Can you work these out from the model? Positions are in its coordinate system, mm. A direction names the side the tool comes from. Round coordinates to 2 decimals unless told otherwise and drop trailing zeros. Loops run counter-clockwise (first coordinate to the right, second up) from the corner with the lowest first, then second, coordinate; pieces in that order, holes last. Notation, with made-up numbers: (-38.75, 70) -> (-15.75, 70) arc R21 ccw to (-15.75, 83) -> close; hole circle Ø7 at (27.5, 49.25). An arc over 180 degrees is marked (long way). Write item = value, one per line.
Autodesk Inventor part; units mm, degrees
ref_plane "YZ Plane" through (0, 0, 0) normal (1, 0, 0) x (0, 1, 0)
ref_plane "XZ Plane" through (0, 0, 0) normal (0, 1, 0) x (-1, 0, 0)
ref_plane "XY Plane" through (0, 0, 0) normal (0, 0, 1) x (1, 0, 0)
sketch "Sketch1" plane through (0, 0, 0) normal (0, 0, 1) x (1, 0, 0)
  line L0 (0, 0) -> (-50, 0) construction
  line L1 (-50, 0) -> (-50, 10)
  line L2 (-50, 0) -> (-50, -10)
  line L3 (-50, -10) -> (-30, -10)
  line L4 (-30, -10) -> (15, -37.5)
  line L5 (-50, 10) -> (-30, 10)
  line L6 (-30, 10) -> (15, 37.5)
  line L7 (15, 37.5) -> (15, -37.5)
  line L8 (0, 0) -> (15, 0) construction
  line L9 (0, 17.5) -> (0, -17.5) construction
  line L10 (-30, 10) -> (40, 10)
  line L11 (-30, -10) -> (40, -10)
  line L12 (40, 10) -> (40, -10)
  circle A0 centre (35, 0) radius 2.25
  circle A1 centre (15, 0) radius 2.25
  line L13 (35, 2.25) -> (15, 2.25)
  line L14 (15, -2.25) -> (35, -2.25)
  point P0 (-40, 0)
  point P1 (40, 0)
  point P2 (15, -10)
  point P3 (15, 10)
  point P4 (-20, 0)
  dimension "d0" = 20
  dimension "d1" = 65
  dimension "d2" = 50
  dimension "d4" = 20
  dimension "d5" = 75
  dimension "d6" = 35
  dimension "d9" = 40
  dimension "d21" = 25
  dimension "d22" = 5
  dimension "d23" = 4.5
  dimension "d30" = 20
extrude "Extrusion1" add sketch "Sketch1" along normal blind 5 contours L1 L5 L10 L7 A1 L11 L3 L2 | L6 L7 L10 | L11 L7 L4 | L7 A1 picked at (13.9746, 0.6255)
hole "Hole1" at (0, 17.5, 0) at (0, -17.5, 0) at (-40, 0, 0) at (0, 0, 0) at (-20, 0, 0) direction (0, 0, 1) diameter 4.5 end through all counterbore diameter 8 counterbore depth 2
fillet "Fillet1" radius 20 2 edges at (-30, 10, 2.5) (-30, -10, 2.5)
chamfer "Chamfer1" distance 2 angle 45 2 edges at (-50, 10, 2.5) (-50, -10, 2.5)
chamfer "Chamfer3" distance 4 angle 45 4 edges at (-5.0992, 25.2172, 0) (-41.8137, 10, 0) (-41.8137, -10, 0) (-5.0992, -25.2172, 0)
properties part number "Y Axis Bearing Holder_3DPrint"
1. For faces 4 (the flat face through (-43, 8, 2)), 5 (the flat face through (-11, 0, 0)), 6 (the flat face through (-43, -8, 2)), 7 (the flat face through (-18, 2, 2)), 8 (the flat face through (-5.381, 25.045, 4.493)), which set-ups out of +Z, -Z, +X, -X, +Y, -Y let a thin tool reach every point of the face, with its end or its side?
Entries:
face_4 = -Z, -X, +Y
face_5 = -Z, +X, -X, +Y, -Y
face_6 = -Z, -X, -Y
face_7 = -Z
face_8 = +Z, -Z, -X, +Y
2. Suppose I cut it at D-D, the plane y = 1. List the corners of the cut face in (x, z) for me, and give its area (3 significant figures).
Entries:
outline = (-50, 0) -> (-43.87, 0) -> (-43.87, 2) -> (-42.02, 2) -> (-42.02, 5) -> (-50, 5) -> close; (-37.98, 2) -> (-36.13, 2) -> (-36.13, 0) -> (-23.87, 0) -> (-23.87, 2) -> (-22.02, 2) -> (-22.02, 5) -> (-37.98, 5) -> close; (-17.98, 2) -> (-16.13, 2) -> (-16.13, 0) -> (-3.87, 0) -> (-3.87, 2) -> (-2.02, 2) -> (-2.02, 5) -> (-17.98, 5) -> close; (2.02, 2) -> (3.87, 2) -> (3.87, 0) -> (15, 0) -> (15, 5) -> (2.02, 5) -> close
area = 242 mm²
3. I'm going to push flat-ended pins straight in: pin 1 (1 mm diameter, centred on x = -9.5, z = 2, fed in from -Y); pin 2 (4 mm diameter, centred on x = -1.5, y = 17, fed in from -Z); pin 3 (2 mm diameter, centred on x = -21.5, z = 1.5, fed in from +Y). Where does each tip first touch, or does it pass through?
Entries:
pin_1 = -20.84
pin_2 = 2
pin_3 = 13.59
4. Suppose I cut it at A-A, the plane x = -40. List the corners of the cut face in (y, z) for me, and give its area (3 significant figures).
Entries:
outline = (-10, 4) -> (-6, 0) -> (-4, 0) -> (-4, 2) -> (-2.25, 2) -> (-2.25, 5) -> (-10, 5) -> close; (2.25, 2) -> (4, 2) -> (4, 0) -> (6, 0) -> (10, 4) -> (10, 5) -> (2.25, 5) -> close
area = 54.5 mm²
5. Suppose I cut it at C-C, the plane y = -17.5. List the corners of the cut face in (x, z) for me.
Entries:
outline = (-17.73, 4) -> (-10.06, 0) -> (-4, 0) -> (-4, 2) -> (-2.25, 2) -> (-2.25, 5) -> (-17.73, 5) -> close; (2.25, 2) -> (4, 2) -> (4, 0) -> (15, 0) -> (15, 5) -> (2.25, 5) -> close
6. I need wall thicknesses on line 1 (X direction, y = 0, z = 1.3); line 2 (X direction, y = 17.5, z = 1.5); line 3 (Y direction, x = 0, z = 0.9). Which ranges of each line are inside material? Lowest first, please. Write a range as [from, to].
Entries:
line_1 = [-50, -44], [-36, -24], [-16, -4], [4, 15]
line_2 = [-12.93, -4], [4, 15]
line_3 = [-24.7, -21.5], [-13.5, -4], [4, 13.5], [21.5, 24.7]
7. We'd pull the mould along Y, two halves only. Please class faces 1 (the flat face through (-49, -9, 4)), 2 (the flat face through (-11, 1, 5)), 3 (the flat face through (2, 2, 2)): released by +Y, released by -Y, zero draft, split by the parting line, or undercut.
Entries:
face_1 = released by -Y
face_2 = zero draft
face_3 = undercut
8. Suppose I cut it at B-B, the plane x = 0. Count the separate pieces of the cut face and the enclosed holes in it, and give its area (3 significant figures).
Entries:
separate_pieces = 4
enclosed_holes = 0
area = 176 mm²
